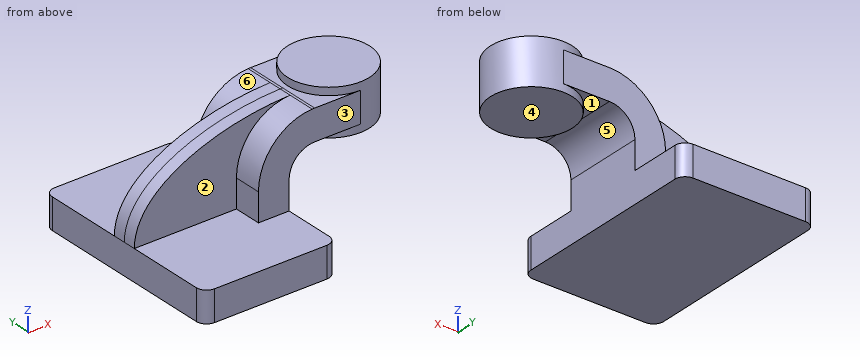
from build123d import *

# Parameters (mm, degrees)
F1_DEPTH = 63.5
F0_W     = 25.4
F0_H     = 19.05
F2_DEPTH = 25.4
F3_DEPTH = 7.9375
F5_R     = 6.35


# Not quite as in the source:
# - a feature names something its author has since deleted; it is built from what else it names


with BuildPart() as f1:
    # F0 (on Front) → F1 (new body, symmetric)
    with BuildSketch(Plane.XZ):
        Polygon((-41.275, 9.525), (-41.275, -9.525), (41.275, -9.525), (41.275, 9.525), (22.225, 9.525), align=None)
    extrude(amount=F1_DEPTH, both=True)

    # F0 (on Front) → F2 (join, symmetric)
    with BuildSketch(Plane.XZ):
        with BuildLine():
            Line((22.225, 9.525), (41.275, 9.525))
            Line((41.275, 9.525), (41.275, 27.0002))
            ThreePointArc((41.275, 27.0002), (45.9246798487, 38.2255201513), (57.15, 42.8752))
            Line((57.15, 42.8752), (60.325, 42.8752))
            Line((60.325, 42.8752), (60.325, 61.9252))
            Line((60.325, 61.9252), (57.15, 61.9252))
            add(Edge.make_bspline(
                [(55.607749268, 61.89113131), (56.1221853633, 61.9046338014), (56.6362918319, 61.9159921928), (57.15, 61.9252)],
                knots=[110.2962801392, 110.2962801392, 110.2962801392, 110.2962801392, 111.5045361635, 111.5045361635, 111.5045361635, 111.5045361635], degree=3))
            ThreePointArc((55.607749268, 61.89113131), (31.9149179532, 51.1444800491), (22.225, 27.0002))
            Line((22.225, 27.0002), (22.225, 9.525))
        make_face()
        with Locations((73.025, 52.4002)):
            Rectangle(F0_W, F0_H)
    extrude(amount=F2_DEPTH, both=True)

    # F0 (on Front) → F3 (join, symmetric)
    with BuildSketch(Plane.XZ):
        with BuildLine():
            add(Edge.make_bspline(
                [(-41.275, 9.525), (-41.060178382, 41.5590820395), (8.6471825165, 60.6585493514), (55.607749268, 61.89113131)],
                knots=[0, 0, 0, 0, 110.2962801392, 110.2962801392, 110.2962801392, 110.2962801392], degree=3))
            Line((-41.275, 9.525), (22.225, 9.525))
            Line((22.225, 9.525), (22.225, 27.0002))
            ThreePointArc((22.225, 27.0002), (31.9149179532, 51.1444800491), (55.607749268, 61.89113131))
        make_face()
    extrude(amount=F3_DEPTH, both=True)

    # F0 (on Front) → F4 (revolve)
    with BuildSketch(Plane.XZ):
        Polygon((85.725, 66.675), (85.725, 61.9252), (85.725, 42.8752), (85.725, 38.1), (111.125, 38.1), (111.125, 66.675), align=None)
    revolve(axis=Axis((85.725, 0, 52.3875), (0, 0, -1)))

    # F5
    f5_edges = [f1.edges().sort_by_distance(p)[0] for p in [
        (41.275, -63.5, 0),
        (41.275, 63.5, 0),
        (-41.275, -63.5, 0),
        (-41.275, 63.5, 0),
    ]]
    fillet(f5_edges, radius=F5_R)


solid = f1.part
The listing builds one solid part. Answer for the finished solid, in the listing's coordinates (mm). Face numbers are marked on the shaded views. A direction names the side the tool comes from. Coordinates: 2 decimals unless noted, no trailing zeros. Write each loop counter-clockwise with the first axis right and the second up, starting at its lowest first coordinate (ties: lowest second). Pieces come first, ordered by that corner, then holes. Notation, with made-up numbers: (83.25, 84) -> (106.25, 84) arc R13 cw to (106.25, 105) -> close; hole circle Ø8 at (-3, 4). An arc over 180 degrees is marked (long way). One line per question, with ' | ' between items.
1. For a pull along X with two mould halves and no side action, classify the marked faces 4, 5 and 6 as released by +X, released by -X, zero draft, split by the parting line, or undercut.
Verdict:
face 4: zero draft | face 5: undercut | face 6: released by -X
2. Straight lines are drawn through the part: line 1 (Z direction, x = 84.5, y = 10.5) (3 decimals); line 2 (Y direction, x = -9.5, z = 22.5); line 3 (X direction, y = 3, z = 8) (3 decimals). For each, find the intervals that lie inside material, in ascending order.
Verdict:
line 1: z = 38.1 to 66.675 | line 2: y = -7.94 to 7.94 | line 3: x = -41.275 to 41.275
3. Section A-A (z = -3.5) is taken. Determine the outline of the cut face in (x, y) (3 decimals).
Verdict:
outline: (-41.275, -57.15) arc R6.35 ccw to (-34.925, -63.5) -> (34.925, -63.5) arc R6.35 ccw to (41.275, -57.15) -> (41.275, 57.15) arc R6.35 ccw to (34.925, 63.5) -> (-34.925, 63.5) arc R6.35 ccw to (-41.275, 57.15) -> close
4. Which of the six approach directions +Z, -Z, +X, -X, +Y, -Y give full straight-line access (tool end or side, diameter ignored) to the marked faces 1, 2 and 3?
Verdict:
face 1: -Z | face 2: +Z, -X, -Y | face 3: +Z, +X, -X, -Y
5. Section B-B (y = -50) is taken. Determine the outline of the cut face in (x, z) (3 decimals), and give its area (3 significant figures).
Verdict:
outline: (-41.275, -9.525) -> (41.275, -9.525) -> (41.275, 9.525) -> (-41.275, 9.525) -> close | area: 1,570 mm^2
6. Given pin 1 Ø8.5 at (y, z) = (18, 17.5) entering from -X (3 decimals); pin 2 Ø6 at (y, z) = (-12.5, 22) entering from +X (3 decimals); pin 3 Ø16.5 at (x, y) = (-19.5, 49) entering from +Z (3 decimals), each flat-ended and moving along its own axis, determine where each tip first touches the part or whether it passes through.
Verdict:
pin 1: stops at x = 22.225 | pin 2: stops at x = 41.275 | pin 3: stops at z = 9.525
